Read the model definition and answer for the solid it produces. Units are mm, in the model's axes. Coordinates: 2 decimals unless noted, no trailing zeros. Order: outer loops, then holes, each group sorted by start corner. A loop starts at its lowest first (then second) coordinate and runs counter-clockwise, first axis right, second up.
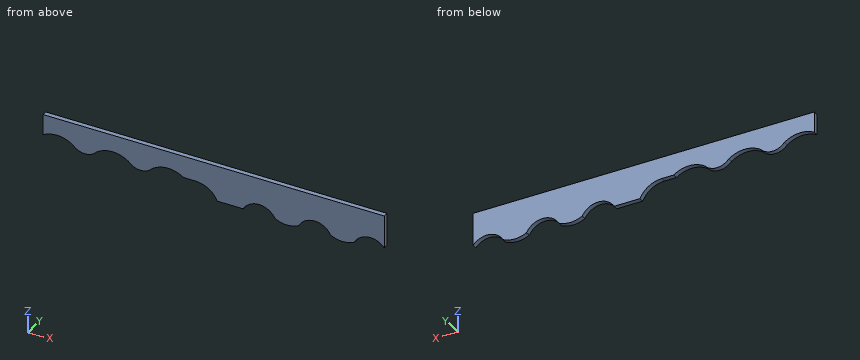
```python
from build123d import *

# Parameters (mm, degrees)
BOSS_EXTRUDE1_DEPTH = 2
SKETCH3_W           = 150.539703927
SKETCH3_H           = 27.267854048
CUT_EXTRUDE2_DEPTH  = 2
FILLET2_R           = 10


with BuildPart() as part:
    # Sketch1 → Boss-Extrude1 (new body)
    with BuildSketch(Plane(origin=(0, 0, 0), x_dir=(1, 0, 0), z_dir=(0, 1, 0))):
        with BuildLine():
            Line((-52.137643745, -8.908278482), (-52.137643745, -18.874998482))
            Line((-52.137643745, -18.874998482), (89.612643745, -18.874998482))
            Line((89.612643745, -18.874998482), (89.612643745, -3.176759435))
            ThreePointArc((89.612643745, -3.176759435), (83.375, -7), (77.137356255, -3.176759435))
            ThreePointArc((77.137356255, -3.176759435), (71.9, -1.832537182), (66.662643745, -3.176759435))
            ThreePointArc((66.662643745, -3.176759435), (60.425, -7), (54.187356255, -3.176759435))
            ThreePointArc((54.187356255, -3.176759435), (48.95, -1.832537182), (43.712643745, -3.176759435))
            ThreePointArc((43.712643745, -3.176759435), (37.475, -7), (31.237356255, -3.176759435))
            Line((31.237356255, -3.176759435), (19.762356255, -3.176759435))
            Line((19.762356255, -3.176759435), (19.762356255, -8.908278482))
            Line((19.762356255, -8.908278482), (6.237643745, -8.908278482))
            ThreePointArc((6.237643745, -8.908278482), (0, -10.875), (-6.237643745, -8.908278482))
            ThreePointArc((-6.237643745, -8.908278482), (-11.475, -6.552640597), (-16.712356255, -8.908278482))
            ThreePointArc((-16.712356255, -8.908278482), (-22.95, -10.875), (-29.187643745, -8.908278482))
            ThreePointArc((-29.187643745, -8.908278482), (-34.425, -6.552640597), (-39.662356255, -8.908278482))
            ThreePointArc((-39.662356255, -8.908278482), (-45.9, -10.875), (-52.137643745, -8.908278482))
        make_face()
    extrude(amount=BOSS_EXTRUDE1_DEPTH)

    # Sketch3 → Cut-Extrude2 (cut)
    with BuildSketch(Plane(origin=(0, 2, 0), x_dir=(1, 0, 0), z_dir=(0, 1, 0))):
        with Locations((17.759945942, -9.959763718)):
            Rectangle(SKETCH3_W, SKETCH3_H)
        with BuildLine():
            Line((89.112643745, -18.374998482), (89.112643745, -4.83005634))
            ThreePointArc((89.112643745, -4.83005634), (82.598017349, -7.459644627), (76.765134062, -3.543962794))
            ThreePointArc((76.765134062, -3.543962794), (71.9, -2.332537182), (67.034865938, -3.543962794))
            ThreePointArc((67.034865938, -3.543962794), (60.425, -7.5), (53.815134062, -3.543962794))
            ThreePointArc((53.815134062, -3.543962794), (48.95, -2.332537182), (44.084865938, -3.543962794))
            ThreePointArc((44.084865938, -3.543962794), (37.550754129, -7.499617411), (30.938071053, -3.676759435))
            Line((30.938071053, -3.676759435), (20.262356255, -3.676759435))
            Line((20.262356255, -3.676759435), (20.262356255, -9.408278482))
            Line((20.262356255, -9.408278482), (6.393349749, -9.408278482))
            ThreePointArc((6.393349749, -9.408278482), (-0.109944429, -11.374468657), (-6.574017094, -9.282937264))
            ThreePointArc((-6.574017094, -9.282937264), (-11.475, -7.052640597), (-16.375982906, -9.282937264))
            ThreePointArc((-16.375982906, -9.282937264), (-22.95, -11.375), (-29.524017094, -9.282937264))
            ThreePointArc((-29.524017094, -9.282937264), (-34.425, -7.052640597), (-39.325982906, -9.282937264))
            ThreePointArc((-39.325982906, -9.282937264), (-45.402501157, -11.364115447), (-51.637643745, -9.821917799))
            Line((-51.637643745, -9.821917799), (-51.637643745, -18.374998482))
            Line((-51.637643745, -18.374998482), (89.112643745, -18.374998482))
        make_face(mode=Mode.SUBTRACT)
    extrude(amount=-CUT_EXTRUDE2_DEPTH, mode=Mode.SUBTRACT)

    # Fillet2
    # the kernel refuses this fillet: 10 mm, written as the material it adds along each edge
    with BuildSketch(Plane(origin=(20.262356255, 2, 9.408278482), x_dir=(-1, 0, 0), z_dir=(0, -1, 0))) as fillet2_piece_1:
        with BuildLine():
            CenterArc((9.043233401, 10), FILLET2_R, 205.267698006, 64.732301994)
            Line((0, 5.731519047), (-0.180864668, 5.646149428))
            ThreePointArc((-0.180864668, 5.646149428), (-0.2, 2.865759523), (-0.2, 0))
            Line((-0.2, 0), (0, -0.2))
            Line((0, -0.2), (9.043233401, -0.2))
            Line((9.043233401, -0.2), (9.043233401, 0))
        make_face()
    extrude(amount=2)


solid = part.part
```
1) A cutting plane is placed at A-A, the plane y = 0.9. Determine the outline of the cut face in (x, z) (3 decimals).
A:
outline: (-51.638, 9.822) arc R11.375 cw to (-39.326, 9.283) arc R6.5 ccw to (-29.524, 9.283) arc R11.375 cw to (-16.376, 9.283) arc R6.5 ccw to (-6.574, 9.283) arc R11.375 cw to (6.393, 9.408) - (11.219, 9.408) arc R10 cw to (20.262, 3.677) - (30.938, 3.677) arc R7.5 cw to (44.085, 3.544) arc R10.375 ccw to (53.815, 3.544) arc R7.5 cw to (67.035, 3.544) arc R10.375 ccw to (76.765, 3.544) arc R7.5 cw to (89.113, 4.83) - (89.113, 18.375) - (-51.638, 18.375) - close
2) Flat-ended cylindrical pins translate along their axes: pin 1 Ø1 at (x, y) = (24, 1) entering from -Z; pin 2 Ø8 at (x, z) = (70, 7) entering from -Y; pin 3 Ø0.6 at (x, y) = (8.5, 1.5) entering from -Z. Find the tip coordinate at first contact, or state that the pin passes through.
A:
pin 1: stops at z = 3.68
pin 2: stops at y = 0
pin 3: stops at z = 9.41
3) Straight lines are drawn through the part: line 1 (X direction, y = 0.7, z = 6.25); line 2 (X direction, y = 0.2, z = 6) (3 decimals); line 3 (Z direction, x = 40, y = 0.95) (3 decimals). For each, find the intervals that lie inside material, in ascending order.
A:
line 1: x = 18.51 to 33.33, 41.62 to 56.28, 64.57 to 79.23, 87.52 to 89.11
line 2: x = 18.739 to 32.975, 41.975 to 55.925, 64.925 to 78.875, 87.875 to 89.113
line 3: z = 7.062 to 18.375
4) A cutting plane is placed at B-B, the plane x = 21.5. Determine the outline of the cut face in (y, z) (3 decimals).
A:
outline: (0, 3.677) - (2, 3.677) - (2, 18.375) - (0, 18.375) - close
5) A cutting plane is placed at C-C, the plane x = -23.5. Determine the outline of the cut face in (y, z) (3 decimals), and give its area (3 significant figures).
A:
outline: (0, 11.362) - (2, 11.362) - (2, 18.375) - (0, 18.375) - close
area: 14.0 mm2
